from build123d import *

# Parameters (mm, degrees)
EXTRUDE_1_DEPTH          = 34
SKETCH_2_R               = 1
CUT_EXTRUDE_4_DEPTH      = 35
CUT_EXTRUDE_4_DEPTH_BACK = 30
SKETCH_3_W               = 20
SKETCH_3_H               = 30
CUT_EXTRUDE_5_DEPTH      = 30
CUT_EXTRUDE_5_DEPTH_BACK = 30


with BuildPart() as part:
    # 草圖1 → 填料-伸長1 (new body)
    with BuildSketch(Plane.XY):
        with BuildLine():
            Line((-35, 5), (35, 5))
            ThreePointArc((35, 5), (40, 0), (35, -5))
            Line((35, -5), (-35, -5))
            ThreePointArc((-35, -5), (-40, 0), (-35, 5))
        make_face()
    extrude(amount=EXTRUDE_1_DEPTH)

    # 草圖2 → 除料-伸長4 (cut, two sides)
    with BuildSketch(Plane.XY) as cut_extrude_4_sk:
        with Locations((-35, 0)):
            Circle(SKETCH_2_R)
        with Locations((35, 0)):
            Circle(SKETCH_2_R)
    extrude(amount=CUT_EXTRUDE_4_DEPTH, mode=Mode.SUBTRACT)
    extrude(cut_extrude_4_sk.sketch, amount=-CUT_EXTRUDE_4_DEPTH_BACK, mode=Mode.SUBTRACT)

    # 草圖3 → 除料-伸長5 (cut, two sides)
    with BuildSketch(Plane(origin=(0, 0, 0), x_dir=(1, 0, 0), z_dir=(0, 1, 0))) as cut_extrude_5_sk:
        with Locations((-30, -17)):
            Rectangle(SKETCH_3_W, SKETCH_3_H)
        with Locations((30, -17)):
            Rectangle(SKETCH_3_W, SKETCH_3_H)
    extrude(amount=CUT_EXTRUDE_5_DEPTH, mode=Mode.SUBTRACT)
    extrude(cut_extrude_5_sk.sketch, amount=-CUT_EXTRUDE_5_DEPTH_BACK, mode=Mode.SUBTRACT)


solid = part.part
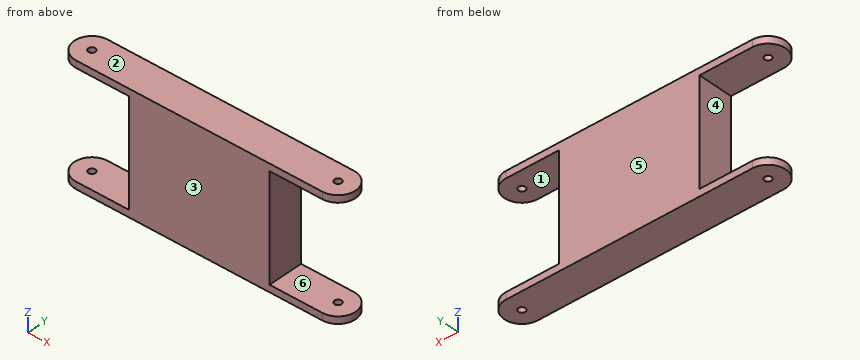
Check sheet for the modelled part. Datum: model origin and axes. Units: mm. Face numbers are marked on the shaded views. A direction names the side the tool comes from. Give positions to 0.01 mm unless a question says otherwise; leave off trailing zeros. Write each loop counter-clockwise with the first axis right and the second up, starting at its lowest first coordinate (ties: lowest second). Pieces come first, ordered by that corner, then holes. Notation, with made-up numbers: (16.25, 55) -> (42.25, 55) arc R10 ccw to (42.25, 65) -> close; hole circle Ø10 at (-34, -24). An arc over 180 degrees is marked (long way). Use one line per item in the form item = value. Start each with the question number.
1. Access from +Z, -Z, +X, -X, +Y, -Y to the whole of each face (thin tool, end or side, straight path). Record for the marked faces 4, 5 and 6.
2. Thickness scan on line 1 along X through (y, z) = (0, 32.85); line 2 along Y through (x, z) = (35, 1.2); line 3 along Z through (x, y) = (29, -3). Record the ranges inside material, lowest first. Write a range as from..to.
3. Section check A-A (y = 0). Record the cut outline in (x, z).
4. Section check C-C (y = 4). Record the cut outline in (x, z).
5. Go/stop test with flat-tipped pins: P1, Ø3, axis at x = 35, y = 0, coming from the -Z side; P2, Ø1.2, axis at x = -35, y = 0, coming from the +Z side; P3, Ø6, axis at y = 1.5, z = 20.5, coming from the +X side. Record where each tip stops, or that it passes through.
6. Mould release check, pull along Z, two halves, no side actions. Record for the marked faces 1, 2 and 3: pulls with the +Z half, pulls with the -Z half, needs draft (parallel to the pull), parting line crosses it, or undercut.
7. Section check B-B (x = 30). Record the cut outline in (y, z), and give its area (3 significant figures).
8. Section check D-D (z = 16). Record the cut outline in (x, y), and give its area (3 significant figures).
Conclusion:
q1.face_4 = -X, +Y, -Y
q1.face_5 = +Z, -Z, +X, -X, +Y
q1.face_6 = +X, +Y, -Y
q2.line_1 = -40..-36, -34..34, 36..40
q2.line_2 = -5..-1, 1..5
q2.line_3 = 0..2, 32..34
q3.outline = (-40, 0) -> (-36, 0) -> (-36, 2) -> (-40, 2) -> close; (-40, 32) -> (-36, 32) -> (-36, 34) -> (-40, 34) -> close; (-34, 0) -> (34, 0) -> (34, 2) -> (20, 2) -> (20, 32) -> (34, 32) -> (34, 34) -> (-34, 34) -> (-34, 32) -> (-20, 32) -> (-20, 2) -> (-34, 2) -> close; (36, 0) -> (40, 0) -> (40, 2) -> (36, 2) -> close; (36, 32) -> (40, 32) -> (40, 34) -> (36, 34) -> close
q4.outline = (-38, 0) -> (38, 0) -> (38, 2) -> (20, 2) -> (20, 32) -> (38, 32) -> (38, 34) -> (-38, 34) -> (-38, 32) -> (-20, 32) -> (-20, 2) -> (-38, 2) -> close
q5.P1 = 0
q5.P2 = through
q5.P3 = 20
q6.face_1 = undercut
q6.face_2 = pulls with the +Z half
q6.face_3 = needs draft
q7.outline = (-5, 0) -> (5, 0) -> (5, 2) -> (-5, 2) -> close; (-5, 32) -> (5, 32) -> (5, 34) -> (-5, 34) -> close
q7.area = 40.0 mm²
q8.outline = (-20, -5) -> (20, -5) -> (20, 5) -> (-20, 5) -> close
q8.area = 400 mm²
